Here's how the part is built. I have some questions about the finished solid (model axes, mm). Give positions to 0.01 mm unless a question says otherwise; leave off trailing zeros. Write each loop counter-clockwise with the first axis right and the second up, starting at its lowest first coordinate (ties: lowest second). Pieces come first, ordered by that corner, then holes. Notation, with made-up numbers: (-14, 87.5) -> (19, 87.5) arc R37 ccw to (19, 123.5) -> close; hole circle Ø3 at (79, 58). An arc over 180 degrees is marked (long way). Use one line per item in the form item = value.
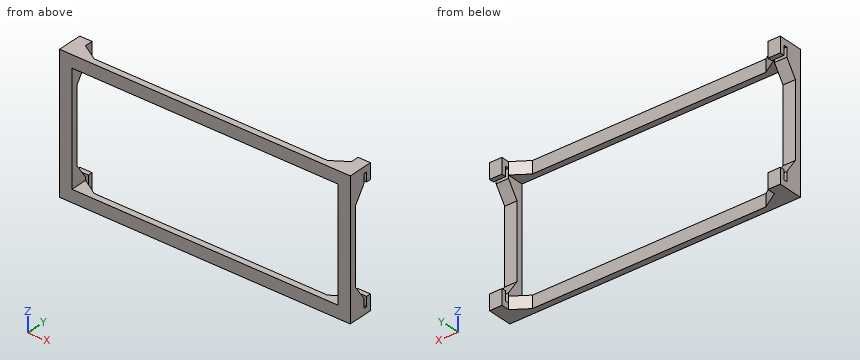
```python
from build123d import *

# Parameters (mm, degrees)
SKETCH_1_W       = 94
SKETCH_1_H       = 44
SKETCH_1_W_2     = 86
SKETCH_1_H_2     = 36
EXTRUDE_2_DEPTH  = 2
EXTRUDE_3_DEPTH  = 4
EXTRUDE_4_DEPTH  = 4
EXTRUDE_5_DEPTH  = 4
EXTRUDE_6_DEPTH  = 4
EXTRUDE_7_DEPTH  = 4
EXTRUDE_8_DEPTH  = 4
EXTRUDE_9_DEPTH  = 4
EXTRUDE_10_DEPTH = 4


with BuildPart() as part:
    # Эскиз1 → Бобышка-Вытянуть2 (new body)
    with BuildSketch(Plane(origin=(0, 0, 0), x_dir=(1, 0, 0), z_dir=(0, 1, 0))):
        Rectangle(SKETCH_1_W, SKETCH_1_H)
        Rectangle(SKETCH_1_W_2, SKETCH_1_H_2, mode=Mode.SUBTRACT)
    extrude(amount=EXTRUDE_2_DEPTH)

    # Эскиз2 → Бобышка-Вытянуть3 (add)
    with BuildSketch(Plane(origin=(47, 0, 0), x_dir=(0, 0, -1), z_dir=(1, 0, 0))):
        Polygon((-22, 8), (-22, 2), (-17, 2), (-17, 5.4), (-20, 5.4), (-20, 6.5), (-17, 6.5), (-17, 8), align=None)
        Polygon((-17, 5.4), (-17, 2), (-12, 2), align=None)
    extrude(amount=-EXTRUDE_3_DEPTH)

    # Эскиз3 → Бобышка-Вытянуть4 (add)
    with BuildSketch(Plane(origin=(47, 0, 0), x_dir=(0, 0, -1), z_dir=(1, 0, 0))):
        Polygon((17, 2), (22, 2), (22, 8), (17, 8), (17, 6.5), (20, 6.5), (20, 5.4), (17, 5.4), align=None)
        Polygon((12, 2), (17, 2), (17, 5.4), align=None)
    extrude(amount=-EXTRUDE_4_DEPTH)

    # Эскиз4 → Бобышка-Вытянуть5 (add)
    with BuildSketch(Plane.ZY.offset(47)):
        Polygon((-22, 8), (-22, 2), (-17, 2), (-17, 5.4), (-20, 5.4), (-20, 6.5), (-17, 6.5), (-17, 8), align=None)
        Polygon((-17, 5.4), (-17, 2), (-12, 2), align=None)
    extrude(amount=-EXTRUDE_5_DEPTH)

    # Эскиз5 → Бобышка-Вытянуть6 (add)
    with BuildSketch(Plane.ZY.offset(47)):
        Polygon((12, 2), (17, 2), (17, 5.4), align=None)
        Polygon((17, 2), (22, 2), (22, 8), (17, 8), (17, 6.5), (20, 6.5), (20, 5.4), (17, 5.4), align=None)
    extrude(amount=-EXTRUDE_6_DEPTH)

    # Эскиз6 → Бобышка-Вытянуть7 (add)
    with BuildSketch(Plane.XY.offset(22)):
        Polygon((-43, 2), (-43, 5.4), (-37.433571672, 2), align=None)
    extrude(amount=-EXTRUDE_7_DEPTH)

    # Эскиз7 → Бобышка-Вытянуть8 (add)
    with BuildSketch(Plane.XY.offset(22)):
        Polygon((43, 2), (43, 5.4), (38, 2), align=None)
    extrude(amount=-EXTRUDE_8_DEPTH)

    # Эскиз8 → Бобышка-Вытянуть9 (add)
    with BuildSketch(Plane(origin=(0, 0, -22), x_dir=(-1, 0, 0), z_dir=(0, 0, -1))):
        Polygon((-43, 2), (-43, 5.4), (-38, 2), align=None)
    extrude(amount=-EXTRUDE_9_DEPTH)

    # Эскиз9 → Бобышка-Вытянуть10 (add)
    with BuildSketch(Plane(origin=(0, 0, -22), x_dir=(-1, 0, 0), z_dir=(0, 0, -1))):
        Polygon((43, 2), (43, 5.4), (37.433571672, 2), align=None)
    extrude(amount=-EXTRUDE_10_DEPTH)


solid = part.part
```
Q1. Will this pin go through, and if not, where does the flat tip stop? pin 1 Ø3 at (x, z) = (-2.5, 19.5) entering from +Y.
Result set:
pin_1 = 2
Q2. I want a section at A-A, the plane x = -4.5. Write out the boundary of the cut face in (y, z), and give its area (3 significant figures).
Result set:
outline = (0, -22) -> (2, -22) -> (2, -18) -> (0, -18) -> close; (0, 18) -> (2, 18) -> (2, 22) -> (0, 22) -> close
area = 16.0 mm2
Q3. I want a section at C-C, the plane y = 4. Write out the boundary of the cut face in (x, z).
Result set:
outline = (-47, -22) -> (-40.71, -22) -> (-40.71, -18) -> (-43, -18) -> (-43, -14.94) -> (-47, -14.94) -> close; (-47, 14.94) -> (-43, 14.94) -> (-43, 18) -> (-40.71, 18) -> (-40.71, 22) -> (-47, 22) -> close; (40.94, -22) -> (47, -22) -> (47, -14.94) -> (43, -14.94) -> (43, -18) -> (40.94, -18) -> close; (40.94, 18) -> (43, 18) -> (43, 14.94) -> (47, 14.94) -> (47, 22) -> (40.94, 22) -> close
Q4. I want a section at B-B, the plane z = 15. Write out the boundary of the cut face in (x, y), and give its area (3 significant figures).
Result set:
outline = (-47, 0) -> (-43, 0) -> (-43, 4.04) -> (-47, 4.04) -> close; (43, 0) -> (47, 0) -> (47, 4.04) -> (43, 4.04) -> close
area = 32.3 mm2
Q5. If I drill on line 1 along X through (y, z) = (1.75, -1); line 2 along Z through (x, y) = (39.5, 2.75), over which ranges is the centre line in solid material (lowest first)? Write a range as from..to.
Result set:
line_1 = -47..-43, 43..47
line_2 = -22..-18, 18..22
